Geometry: final body of the model. Coordinates: model frame, mm. A direction names the side the tool comes from. Give positions to 0.01 mm unless a question says otherwise; leave off trailing zeros. Loops run counter-clockwise (first coordinate to the right, second up) from the corner with the lowest first, then second, coordinate; pieces in that order, holes last. Notation, with made-up numbers: M 42,-38 L 46,-38 A14 ccw 46,-21 Z; hole C 8,48.25 d3. An arc over 180 degrees is marked long. Put each result on its own line as item: value.
```python
from build123d import *

# Parameters (mm, degrees)
SKETCH1_R           = 3.175
BOSS_EXTRUDE1_DEPTH = 9.525
BOSS_EXTRUDE2_DEPTH = 4.1402


with BuildPart() as part:
    # Sketch1 → Boss-Extrude1 (new body)
    with BuildSketch(Plane(origin=(0, 0, 0), x_dir=(1, 0, 0), z_dir=(0, 1, 0))):
        with Locations(Location((0, 0, 0), (0, 0, 270))):  # turned: the seam where the file's is
            Circle(SKETCH1_R)
    extrude(amount=-BOSS_EXTRUDE1_DEPTH)

    # Sketch2 → Boss-Extrude2 (add)
    with BuildSketch(Plane(origin=(0, 0, 0), x_dir=(1, 0, 0), z_dir=(0, 1, 0))):
        Polygon((-3.207902433, 5.55625), (3.207902433, 5.55625), (6.415804866, 0), (3.207902433, -5.55625), (-3.207902433, -5.55625), (-6.415804866, 0), align=None)
    extrude(amount=BOSS_EXTRUDE2_DEPTH)


solid = part.part
```
Item 1: Section B-B on z = -2.5. Output: boundary loops of the cut face in (x, y) (3 decimals).
Output values:
outline: M -4.972,0 L -1.957,0 L -1.957,-9.525 L 1.957,-9.525 L 1.957,0 L 4.972,0 L 4.972,4.14 L -4.972,4.14 Z
Item 2: Section D-D on y = -7. Output: boundary loops of the cut face in (x, z) (3 decimals), then the cut area to 3 significant figures.
Output values:
outline: C 0,0 d6.35
area: 31.7 mm²
Item 3: Section A-A on x = 0. Output: boundary loops of the cut face in (y, z) (3 decimals).
Output values:
outline: M -9.525,-3.175 L 0,-3.175 L 0,-5.556 L 4.14,-5.556 L 4.14,5.556 L 0,5.556 L 0,3.175 L -9.525,3.175 Z
Item 4: Pin query (flat end, axial travel): pin 1 Ø3 at (y, z) = (-3.5, -0.5) entering from +X (3 decimals); pin 2 Ø6 at (x, y) = (-1, -4) entering from -Z (3 decimals); pin 3 Ø1.5 at (x, y) = (-2.5, -7) entering from +Z. Return the tip coordinate at first contact, or that it passes through.
Output values:
pin 1: x = 3.175
pin 2: z = -3.175
pin 3: z = 2.65
Item 5: Section C-C on y = 1. Output: boundary loops of the cut face in (x, z).
Output values:
outline: M -6.42,0 L -3.21,-5.56 L 3.21,-5.56 L 6.42,0 L 3.21,5.56 L -3.21,5.56 Z
Item 6: Line query: probe 1 along Y at (x, z) = (-3, 4.5); probe 2 along X at (y, z) = (-0.5, 1.25); probe 3 along X at (y, z) = (-2.5, 2.75). Output: solid intervals per line, ascending. Write a range as [from, to].
Output values:
probe 1: [0, 4.14]
probe 2: [-2.92, 2.92]
probe 3: [-1.59, 1.59]
Item 7: Set-up query: faces 1 (the flat face through (-3, 0, -3)), 2 (the flat face through (0, 2, -5.556)). Return all of +Z, -Z, +X, -X, +Y, -Y with unobstructed straight access to the full face (end or side cutting, diameter ignored); none if empty.
Output values:
face 1: -Y
face 2: -Z, +X, -X, +Y, -Y
